The listing builds one solid part. Answer for the finished solid, in the listing's coordinates (mm). A direction names the side the tool comes from. Round coordinates to 2 decimals unless told otherwise and drop trailing zeros. Loops run counter-clockwise (first coordinate to the right, second up) from the corner with the lowest first, then second, coordinate; pieces in that order, holes last. Notation, with made-up numbers: (87.25, 73.25) - (108.25, 73.25) arc R26 cw to (108.25, 101.25) - close; hole circle Ø11 at (-14.5, 39.5). An arc over 180 degrees is marked (long way). One line per item, written item: value.
```python
from build123d import *

# Parameters (mm, degrees)
BOSS_EXTRUDE1_DEPTH                          = 4
SKETCH2_W                                    = 70
SKETCH2_H                                    = 3
BOSS_EXTRUDE2_DEPTH                          = 5
CSK_FOR_M2_COUNTERSUNK_FLAT_HEAD_SCR_2_COUNT = 2
CSK_FOR_M2_COUNTERSUNK_FLAT_HEAD_SCR_2_PITCH = 10
SKETCH5_W                                    = 10
SKETCH5_H                                    = 3
CUT_EXTRUDE1_DEPTH                           = 5
FILLET1_R                                    = 2.5
M2_TAPPED_HOLE1_D                            = 1.6
M2_TAPPED_HOLE1_DEPTH                        = 3
BOSS_EXTRUDE3_DEPTH                          = 5
FILLET2_R                                    = 2


with BuildPart() as part:
    # Sketch1 → Boss-Extrude1 (new body)
    with BuildSketch(Plane(origin=(0, 0, 0), x_dir=(1, 0, 0), z_dir=(0, 1, 0))):
        Polygon((-4, 0), (4, 0), (4, 7.5), (7, 7.5), (10, 12), (35, 12), (35, 15), (10, 15), (10, 20), (-10, 20), (-10, 15), (-35, 15), (-35, 12), (-10, 12), (-7, 7.5), (-4, 7.5), align=None)
    extrude(amount=BOSS_EXTRUDE1_DEPTH)

    # Sketch2 → Boss-Extrude2 (add)
    with BuildSketch(Plane(origin=(0, 4, 0), x_dir=(1, 0, 0), z_dir=(0, 1, 0))):
        with Locations((0, 13.5)):
            Rectangle(SKETCH2_W, SKETCH2_H)
    extrude(amount=BOSS_EXTRUDE2_DEPTH)

    # Sketch4 → CSK for M2 Countersunk Flat Head Screw1 (revolve, cut)
    with BuildSketch(Plane(origin=(0, 4, -15), x_dir=(0, 0, 1), z_dir=(1, 0, 0))):
        Polygon((0, 0), (0, 4), (1.1, 4), (1.1, 1.1), (2.2, 0), align=None)
    csk_for_m2_countersunk_flat_head_screw1 = revolve(axis=Axis((0, 10.35, -15), (0, -1, 0)), mode=Mode.SUBTRACT)

    # CSK for M2 Countersunk Flat Head Scr 2: CSK for M2 Countersunk Flat Head Screw1 ×2
    with Locations(*[(0, 0, i * CSK_FOR_M2_COUNTERSUNK_FLAT_HEAD_SCR_2_PITCH) for i in range(1, CSK_FOR_M2_COUNTERSUNK_FLAT_HEAD_SCR_2_COUNT)]):
        add(csk_for_m2_countersunk_flat_head_screw1, mode=Mode.SUBTRACT)

    # Sketch5 → Cut-Extrude1 (cut)
    with BuildSketch(Plane(origin=(0, 9, 0), x_dir=(1, 0, 0), z_dir=(0, 1, 0))):
        with Locations((0, 13.5)):
            Rectangle(SKETCH5_W, SKETCH5_H)
    extrude(amount=-CUT_EXTRUDE1_DEPTH, mode=Mode.SUBTRACT)

    # Fillet1
    fillet1_edges = [part.edges().sort_by_distance(p)[0] for p in [
        (-35, 0, -13.5),
        (35, 0, -13.5),
    ]]
    fillet(fillet1_edges, radius=FILLET1_R)

    # M2 Tapped Hole1
    with Locations(Plane(origin=(0, 0, -15), x_dir=(-1, 0, 0), z_dir=(0, 0, -1))):
        with Locations((30, 4), (15, 4), (-15, 4), (-30, 4)):
            Hole(M2_TAPPED_HOLE1_D / 2, depth=M2_TAPPED_HOLE1_DEPTH)

    # Sketch9 → Boss-Extrude3 (add)
    with BuildSketch(Plane(origin=(0, 4, 0), x_dir=(1, 0, 0), z_dir=(0, 1, 0))):
        Polygon((-7.5, 12), (-5.5, 9), (5.5, 9), (7.5, 12), align=None)
    extrude(amount=BOSS_EXTRUDE3_DEPTH)

    # Fillet2
    fillet2_edges = [part.edges().sort_by_distance(p)[0] for p in [
        (7.5, 6.5, -12),
        (-7.5, 6.5, -12),
        (-4, 2, -7.5),
        (-10, 2, -12),
        (10, 2, -12),
        (4, 2, -7.5),
        (-5, 6.5, -12),
        (5, 6.5, -12),
    ]]
    fillet(fillet2_edges, radius=FILLET2_R)


solid = part.part
```
1) For a pull along X with two mould halves and no side action, classify faces 1 (the flat face through (8, 2, -9)), 2 (the cylindrical face through (14.37, 3.51, -13.48)), 3 (the flat face through (0, 6, -9)) as released by +X, released by -X, zero draft, split by the parting line, or undercut.
Final values:
face 1: released by +X
face 2: undercut
face 3: zero draft
2) Each of these flat-tipped pins is pushed along its axis until it touches: pin 1 Ø1.8 at (x, y) = (30, 4) entering from +Z; pin 2 Ø2.5 at (x, y) = (-0.5, 7) entering from -Z; pin 3 Ø2 at (x, y) = (-22, 6.5) entering from -Z; pin 4 Ø1 at (x, y) = (-15, 4) entering from +Z. Where does it stop, or does it pass through?
Final values:
pin 1: z = -12
pin 2: z = -12
pin 3: z = -15
pin 4: through
3) Consider L1, parallel to Z at x = 0, y = 0.95; L2, parallel to Y at x = -30, z = -13.8; L3, parallel to Z at x = -26, y = 7. Determine where each line is inside the solid, lowest interval first.
Final values:
L1: -20 to -16.1, -13.9 to -6.1, -3.9 to 0
L2: 0 to 3.2, 4.8 to 9
L3: -15 to -12
4) A cutting plane is placed at A-A on x = 0. Give the vertices of the cut face in (y, z).
Final values:
outline: (0, -20) - (4, -20) - (4, -17.2) - (2.9, -16.1) - (0, -16.1) - close; (0, -13.9) - (2.9, -13.9) - (4, -12.8) - (4, -12) - (9, -12) - (9, -9) - (4, -9) - (4, -7.2) - (2.9, -6.1) - (0, -6.1) - close; (0, -3.9) - (2.9, -3.9) - (4, -2.8) - (4, 0) - (0, 0) - close
5) For faces 4 (the flat face through (-4, 2, -3)), 5 (the flat face through (-10, 2, -18)), 6 (the cylindrical face through (4.4, 6.46, -12.57)), determine the directions among +Z, -Z, +X, -X, +Y, -Y from which every point of the face is accessible in a straight line to the end or side of a thin tool.
Final values:
face 4: +Z, -X, +Y, -Y
face 5: -Z, -X, +Y, -Y
face 6: -Z, +Y
6) A cutting plane is placed at B-B on x = 30. Give the vertices of the cut face in (y, z).
Final values:
outline: (0, -15) - (3.2, -15) - (3.2, -12) - (0, -12) - close; (4.8, -15) - (9, -15) - (9, -12) - (4.8, -12) - close
7) A cutting plane is placed at C-C on z = -10.25. Give the vertices of the cut face in (x, y), and give its area (3 significant figures).
Final values:
outline: (-8.83, 0) - (8.83, 0) - (8.83, 4) - (6.33, 4) - (6.33, 9) - (-6.33, 9) - (-6.33, 4) - (-8.83, 4) - close
area: 134 mm2
8) A cutting plane is placed at D-D on x = 22. Give the vertices of the cut face in (y, z).
Final values:
outline: (0, -15) - (9, -15) - (9, -12) - (0, -12) - close
